Solid Edge part; units mm, degrees
sketch "Sketch1" plane through (0, 0, 0) normal (0, -1, 0) x (1, 0, 0)
  line L0 (0, -10) -> (1, -10)
  line L1 (1, -10) -> (1, -0.501)
  line L2 (1, -0.501) -> (0.87, -0.101)
  line L3 (0.87, -0.101) -> (0.87, 0)
  line L4 (0.87, 0) -> (2, 0)
  line L5 (2, 0) -> (1.8863, 1.3)
  line L6 (1.8863, 1.3) -> (0, 1.3)
  dimension "D1" = 0.87
  dimension "D2" = 1
  dimension "D3" = 1.8863
revolve "RevolvedProtrusion1" add sketch "Sketch1" angle 360 about axis through (0, 0, 6) along (0, 0, -1)
fillet "Round_1" radius 0.6 1 edges at (-1.8863, 0, 1.3)
sketch "Sketch2" plane through (0, 0, 0) normal (0, -1, 0) x (1, 0, 0)
  line L0 (-0.25, 1.3) -> (-0.25, 0.8)
  line L1 (-0.25, 0.8) -> (0.25, 0.8)
  line L2 (0.25, 0.8) -> (0.25, 1.3)
  line L3 (0.25, 1.3) -> (-0.25, 1.3)
  dimension "D1" = 0.25
  dimension "D2" = 0.25
extrude "ExtrudedCutout_1" cut sketch "Sketch2" along normal mid plane 4
cosmetic_thread "Thread_1" thread depth 9.499
fillet "Round_2" radius 0.1 1 edges at (-0.87, 0, 0)
chamfer "Chamfer_1" distance 0.0012 angle 30 1 edges at (-1, 0, -10) measured on face at (0.6867, 0.6467, -10)
properties material "Steel"
CAD build for the part. Positions are in the model's coordinates, mm. A direction names the side the tool comes from. Give positions to 0.01 mm unless a question says otherwise; leave off trailing zeros. Loops run counter-clockwise (first coordinate to the right, second up) from the corner with the lowest first, then second, coordinate; pieces in that order, holes last. Notation, with made-up numbers: M -29.75,30 L -22.75,30 A24 ccw -22.75,66 Z; hole C 89.5,-20 d3. An arc over 180 degrees is marked long. Use one line per item in the form item = value.
Item 1: Which spindle directions (+Z, -Z, +X, -X, +Y, -Y) get a long thin tool onto all of the face, cutting with end or side? Do faces 1 (the face through (-0.423, 1.907, 0.538)), 2 (the face through (0, -1, -5)). Say none if no direction does.
Determined:
face_1 = +Z
face_2 = -Z
Item 2: Slice it at D-D (z = 0.5). List the corners of the cut face in (x, y).
Determined:
outline = C 0,0 d3.91
Item 3: Drill centre lines: probe 1 along X at (y, z) = (0, -7); probe 2 along X at (y, z) = (-0.7, 1); probe 3 along Y at (x, z) = (0.6, 0.75). Where is each one in solid material? Low to high. Write a range as from..to.
Determined:
probe_1 = -1..1
probe_2 = -1.72..-0.25, 0.25..1.72
probe_3 = -1.84..1.84
Item 4: Slice it at C-C (z = -4.25). List the corners of the cut face in (x, y), plus the area to 3 significant figures.
Determined:
outline = C 0,0 d2
area = 3.14 mm2
